from build123d import *

# Parameters (mm, degrees)
BOSS_EXTRUDE1_DEPTH = 20
SKETCH3_W           = 30.1
SKETCH3_H           = 5
BOSS_EXTRUDE2_DEPTH = 60
SKETCH4_W           = 5
SKETCH4_H           = 30.1
BOSS_EXTRUDE3_DEPTH = 18.55


with BuildPart() as part:
    # Sketch2 → Boss-Extrude1 (new, symmetric)
    with BuildSketch(Plane(origin=(0, 0, 0), x_dir=(0, 0, -1), z_dir=(1, 0, 0))):
        Polygon((15.05, 0), (-15.05, 0), (-15.05, 23.55), (-10.05, 23.55), (-10.05, 18.55), (-6.5, 15), (-10.05, 11.45), (-10.05, 5), (10.05, 5), (10.05, 11.45), (6.5, 15), (10.05, 18.55), (10.05, 23.55), (15.05, 23.55), align=None)
    extrude(amount=BOSS_EXTRUDE1_DEPTH, both=True)

    # Sketch3 → Boss-Extrude2 (add)
    with BuildSketch(Plane(origin=(20, 0, 0), x_dir=(0, 0, -1), z_dir=(1, 0, 0))):
        with Locations((0, 2.5)):
            Rectangle(SKETCH3_W, SKETCH3_H)
    extrude(amount=BOSS_EXTRUDE2_DEPTH)

    # Sketch4 → Boss-Extrude3 (add)
    with BuildSketch(Plane(origin=(0, 5, 0), x_dir=(1, 0, 0), z_dir=(0, 1, 0))):
        with Locations((22.5, 0)):
            Rectangle(SKETCH4_W, SKETCH4_H)
    extrude(amount=BOSS_EXTRUDE3_DEPTH)


solid = part.part
CAD build for the part. Positions are in the model's coordinates, mm. A direction names the side the tool comes from. Coordinates: 2 decimals unless noted, no trailing zeros. Order: outer loops, then holes, each group sorted by start corner. A loop starts at its lowest first (then second) coordinate and runs counter-clockwise, first axis right, second up.
Item 1: Band-saw the part on C-C on x = 42.5. List the corners of the cut face in (y, z), plus the area to 4 significant figures.
Check sheet entries:
outline: (0, -15.05) - (5, -15.05) - (5, 15.05) - (0, 15.05) - close
area: 150.5 mm2
Item 2: Two-plate mould, pull along Y, no slides. Class faces 1 (the face through (0, 5, 0)), 2 (the face through (7, 9, -15.05)), 3 (the face through (0.3, 16.8, 8.3)): +Y half, -Y half, draft (parallel to the pull), parting line (faces both ways), or undercut.
Check sheet entries:
face 1: undercut
face 2: draft
face 3: +Y half
Item 3: Band-saw the part on A-A on y = 9.25. List the corners of the cut face in (x, z).
Check sheet entries:
outline: (-20, -15.05) - (25, -15.05) - (25, 15.05) - (-20, 15.05) - (-20, 10.05) - (20, 10.05) - (20, -10.05) - (-20, -10.05) - close
Item 4: Band-saw the part on B-B on z = 8.5. List the corners of the cut face in (x, y), plus the area to 3 significant figures.
Check sheet entries:
outline: (-20, 0) - (80, 0) - (80, 5) - (25, 5) - (25, 23.55) - (20, 23.55) - (20, 17) - (-20, 17) - (-20, 13) - (20, 13) - (20, 5) - (-20, 5) - close
area: 753 mm2
Item 5: Band-saw the part on D-D on z = 2. List the corners of the cut face in (x, y).
Check sheet entries:
outline: (-20, 0) - (80, 0) - (80, 5) - (25, 5) - (25, 23.55) - (20, 23.55) - (20, 5) - (-20, 5) - close
Item 6: Drill centre lines: L1, parallel to Z at x = 11, y = 8.5; L2, parallel to X at y = 16.75, z = 9; L3, parallel to X at y = 18.5, z = -7. Where is each one in solid material? Low to high.
Check sheet entries:
L1: z = -15.05 to -10.05, 10.05 to 15.05
L2: x = -20 to 25
L3: x = 20 to 25
Item 7: 3-axis set-ups, long thin cutter, end or side, ignore diameter. For faces 4 (the face through (29, 0, 0)), 5 (the face through (7, 9, 15.05)), 6 (the face through (0.3, 16.8, -8.3)), 7 (the face through (25, 14, 0)), 8 (the face through (0, 8, 10.05)): which of +Z, -Z, +X, -X, +Y, -Y reach the whole face in a straight line?
Check sheet entries:
face 4: +Z, -Z, +X, -X, -Y
face 5: +Z, +X, -X, +Y, -Y
face 6: -X, +Y
face 7: +Z, -Z, +X, +Y
face 8: -X
Item 8: Pin check, flat tips, straight feed: pin 1 Ø5.5 at (y, z) = (14.5, 4.5) entering from +X; pin 2 Ø15 at (x, z) = (47, -3.5) entering from +Y; pin 3 Ø10 at (x, z) = (3.5, 2) entering from +Y. Stop position of each tip, or through.
Check sheet entries:
pin 1: stops at x = 25
pin 2: stops at y = 5
pin 3: stops at y = 15.5
